For this review, take the finished solid that the model builds, in its own axes (mm). Coordinates: 2 decimals unless noted, no trailing zeros. Write each loop counter-clockwise with the first axis right and the second up, starting at its lowest first coordinate (ties: lowest second). Pieces come first, ordered by that corner, then holes. Notation, with made-up numbers: M 14.25,49.5 L 60.25,49.5 A16 cw 60.25,56.5 Z; hole C 11,55 d4. An arc over 180 degrees is marked long. Return JSON: item names as keys, results as strings.
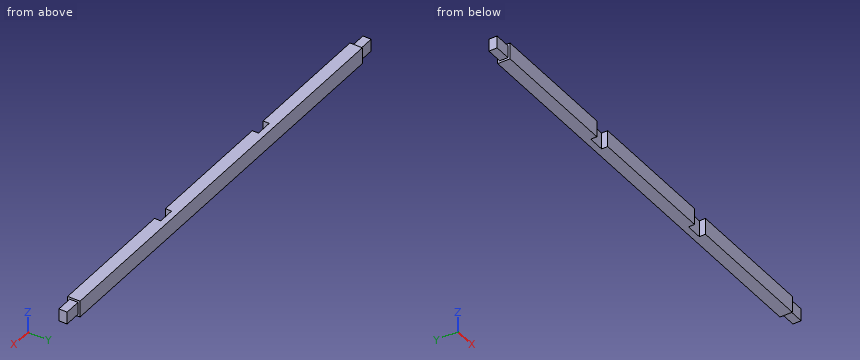
```python
from build123d import *

# Parameters (mm, degrees)
F0_W     = 660.4
F0_H     = 25.4
F1_DEPTH = 9.525
F2_W     = 25.4
F2_H     = 25.4
F3_DEPTH = 9.525
F4_DEPTH = 9.525
F5_W     = 12.7
F5_H     = 19.05
F7_DEPTH = 25.4
F6_W     = 12.7
F6_H     = 19.05
F8_DEPTH = 25.4


with BuildPart() as f1:
    # F0 (on Front) → F1 (new body, symmetric)
    with BuildSketch(Plane.XZ):
        Rectangle(F0_W, F0_H)
    extrude(amount=F1_DEPTH, both=True)

    # F2 (on face) → F3 (cut)
    with BuildSketch(Plane.XZ.offset(9.525)):
        with Locations((-114.3, 0)):
            Rectangle(F2_W, F2_H)
    extrude(amount=-F3_DEPTH, mode=Mode.SUBTRACT)

    # F2 (on face) → F4 (cut)
    with BuildSketch(Plane.XZ.offset(9.525)):
        with Locations((114.3, 0)):
            Rectangle(F2_W, F2_H)
    extrude(amount=-F4_DEPTH, mode=Mode.SUBTRACT)

    # F5 (on face) → F7 (join)
    with BuildSketch(Plane(origin=(-330.2, 0, 0), x_dir=(0, -1, 0), z_dir=(-1, 0, 0))):
        Rectangle(F5_W, F5_H)
    extrude(amount=F7_DEPTH)

    # F6 (on face) → F8 (join)
    with BuildSketch(Plane.YZ.offset(330.2)):
        Rectangle(F6_W, F6_H)
    extrude(amount=F8_DEPTH)


solid = f1.part
```
1. We need section A-A (z = -5). State the section outline as (x, y) points (3 decimals), plus the area to 3 significant figures.
Checks:
{"outline": "M -355.6,-6.35 L -330.2,-6.35 L -330.2,-9.525 L -127,-9.525 L -127,0 L -101.6,0 L -101.6,-9.525 L 101.6,-9.525 L 101.6,0 L 127,0 L 127,-9.525 L 330.2,-9.525 L 330.2,-6.35 L 355.6,-6.35 L 355.6,6.35 L 330.2,6.35 L 330.2,9.525 L -330.2,9.525 L -330.2,6.35 L -355.6,6.35 Z", "area": "12,700 mm2"}
2. We need section B-B (x = 112). State the section outline as (y, z) points (3 decimals).
Checks:
{"outline": "M 0,-12.7 L 9.525,-12.7 L 9.525,12.7 L 0,12.7 Z"}
3. Clearance check with flat-ended pins moving along their axes: pin 1 Ø6.5 at (x, y) = (-346, -1.5) entering from +Z (3 decimals); pin 2 Ø9.5 at (x, z) = (-348, -1) entering from +Y; pin 3 Ø10 at (x, y) = (-343, -2) entering from -Z (3 decimals). State where each tip first meets the part, or that it passes through.
Checks:
{"pin 1": "z = 9.525", "pin 2": "y = 6.35", "pin 3": "z = -9.525"}
4. Wall thickness on L1, parallel to X at y = -6, z = 1; L2, parallel to X at y = -0.75, z = -10.5; L3, parallel to X at y = 3, z = 11: over which ranges is each line inside the solid? List them lowest first. Write a range as from..to.
Checks:
{"L1": "-355.6..-127, -101.6..101.6, 127..355.6", "L2": "-330.2..-127, -101.6..101.6, 127..330.2", "L3": "-330.2..330.2"}
